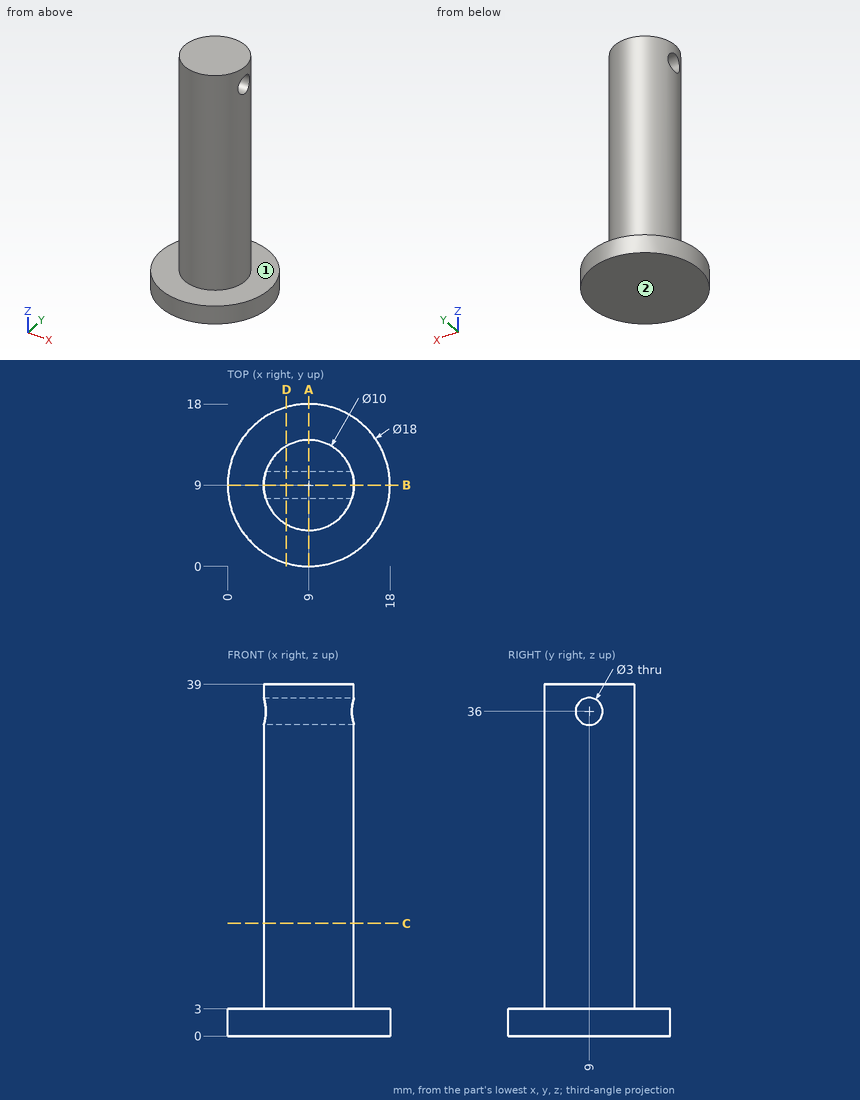
Geometry: see drawing. Coordinates: mm, zero at the bounding-box minimum. A direction names the side the tool comes from. Coordinates: 2 decimals unless noted, no trailing zeros. Order: outer loops, then holes, each group sorted by start corner. A loop starts at its lowest first (then second) coordinate and runs counter-clockwise, first axis right, second up. Notation, with made-up numbers: M -32.75,47.25 L -4.75,47.25 A31 cw -4.75,72.25 Z; hole C 64,73.25 d3. An arc over 180 degrees is marked long. Answer in a Markdown table with one row per item. Add a question column.
Q1. Section query A-A on x = 9. Return the cut outline in (y, z), and give its area (3 significant figures).
Q2. Section query C-C on z = 12.5. Return the cut outline in (x, y), and give its area (3 significant figures).
Q3. Contact query for flat-ended pins moving along their axis: P1, Ø5, axis at x = 4.5, y = 16, coming from the +Z side; P2, Ø2, axis at x = 8.5, z = 33.5, coming from the +Y side; P3, Ø10, axis at y = 9, z = 16, coming from the +X side. Output: stop coordinate, or through.
Q4. Section query B-B on y = 9. Return the cut outline in (x, z), and give its area (3 significant figures).
Q5. Line query: L1, parallel to Y at x = 9, z = 26.5; L2, parallel to Z at x = 7.25, y = 17.25; L3, parallel to Y at x = 8, z = 36. Output: solid intervals per line, ascending.
Q6. Section query D-D on x = 6.5. Return the cut outline in (y, z).
Q7. Reachability of the marked faces 1 and 2 from +Z, -Z, +X, -X, +Y, -Y: full face, straight path, thin tool, end or side. Return the list, or none.
Completed:
| question | item | result |
|---|---|---|
| 1 | outline | M 0,0 L 18,0 L 18,3 L 14,3 L 14,39 L 4,39 L 4,3 L 0,3 Z; hole C 9,36 d3 |
| 1 | area | 407 mm2 |
| 2 | outline | C 9,9 d10 |
| 2 | area | 78.5 mm2 |
| 3 | P1 | stops at z = 3 |
| 3 | P2 | stops at y = 14 |
| 3 | P3 | stops at x = 14 |
| 4 | outline | M 0,0 L 18,0 L 18,3 L 14,3 L 14,34.5 L 4,34.5 L 4,3 L 0,3 Z; M 4,37.5 L 14,37.5 L 14,39 L 4,39 Z |
| 4 | area | 384 mm2 |
| 5 | L1 | y = 4 to 14 |
| 5 | L2 | z = 0 to 3 |
| 5 | L3 | y = 4.1 to 7.5, 10.5 to 13.9 |
| 6 | outline | M 0.35,0 L 17.65,0 L 17.65,3 L 13.33,3 L 13.33,39 L 4.67,39 L 4.67,3 L 0.35,3 Z; hole C 9,36 d3 |
| 7 | face 1 | +Z |
| 7 | face 2 | -Z, +X, -X, +Y, -Y |
